Can you work these out from the drawing? Everything is in mm from the part's minimum corner. Round coordinates to 2 decimals unless told otherwise and drop trailing zeros. Loops run counter-clockwise (first coordinate to the right, second up) from the corner with the lowest first, then second, coordinate; pieces in that order, holes last. Notation, with made-up numbers: (43.5, -5) - (57.5, -5) arc R4 cw to (57.5, 1) - close; hole circle Ø2 at (47.5, 25). An arc over 180 degrees is marked (long way). Answer as CSV lines item,"result". Start each with the question number.
1) Suppose I cut it at B-B, the plane y = 68. Write out the boundary of the cut face in (x, z).
2) Suppose I cut it at A-A, the plane x = 84. Write out the boundary of the cut face in (y, z).
3) Please list where these lines run through material, in increasing order: line 1 along X through (y, z) = (68, 0.75); line 2 along Y through (x, z) = (84, 1.2); line 3 along Y through (x, z) = (85, 2.45).
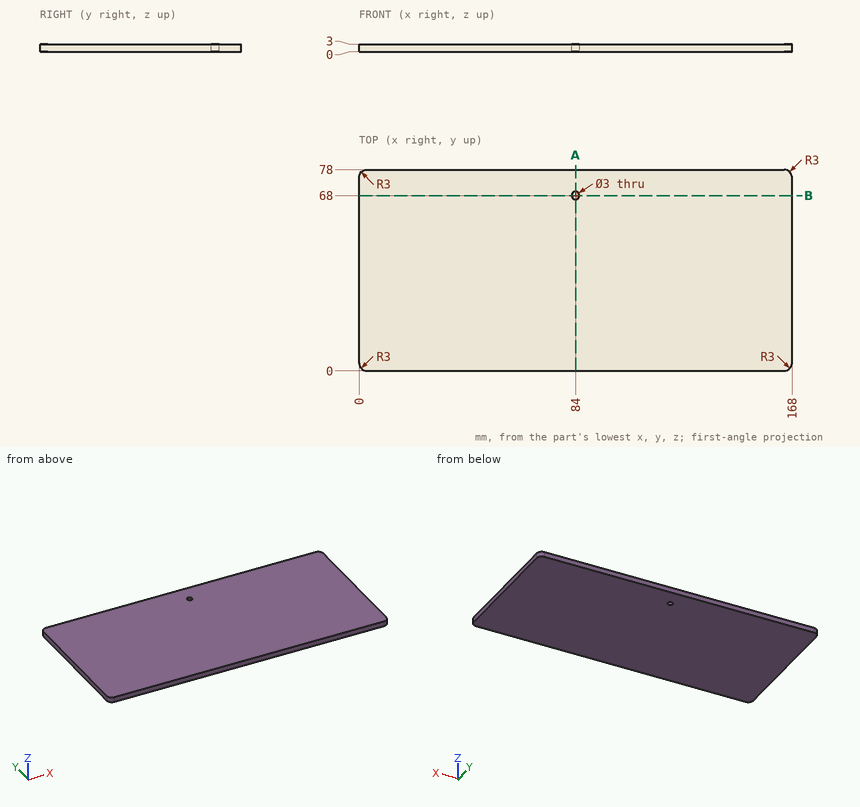
Filled sheet:
1,outline,"(0, 0) - (82.5, 0) - (82.5, 3) - (0, 3) - close; (85.5, 0) - (168, 0) - (168, 3) - (85.5, 3) - close"
2,outline,"(0, 0) - (66.5, 0) - (66.5, 3) - (0, 3) - close; (69.5, 0) - (78, 0) - (78, 3) - (69.5, 3) - close"
3,line 1,"0 to 82.5, 85.5 to 168"
3,line 2,"0 to 66.5, 69.5 to 78"
3,line 3,"0 to 66.88, 69.12 to 78"
